Autodesk Inventor part; units mm, degrees
ref_plane "作業平面1" through (31.0675, 0, 31.152) normal (0, 1, 0) x (0, 0, 1)
ref_plane "YZ Plane" through (0, 0, 0) normal (1, 0, 0) x (0, 1, 0)
ref_plane "XZ Plane" through (0, 0, 0) normal (0, 1, 0) x (-1, 0, 0)
sketch "スケッチ1" plane through (0, 0, 0) normal (0, 1, 0) x (-1, 0, 0)
  line L0 (18, 8) -> (-18, 8) construction
  line L1 (-18, 8) -> (-18, -8) construction
  line L2 (-18, -8) -> (18, -8) construction
  line L3 (18, -8) -> (18, 8) construction
  line L4 (18, 8) -> (-18, -8) construction
  line L5 (-18, 8) -> (18, -8) construction
  circle A0 centre (18, -8) radius 1.1
  circle A1 centre (-18, -8) radius 1.1
  circle A2 centre (-18, 8) radius 1.1
  circle A3 centre (18, -8) radius 2.5
  circle A4 centre (-18, -8) radius 2.5
  circle A5 centre (-18, 8) radius 2.5
  line L6 (18, -10.5) -> (-18, -10.5)
  line L7 (-15.5, 8) -> (-15.5, -8)
  line L8 (-18, -5.5) -> (18, -5.5)
  line L9 (-20.5, -8) -> (-20.5, 8)
  line L10 (-20.5, 0) -> (18, 0) construction
  circle A6 centre (18, 8) radius 1.1
  circle A7 centre (18, 8) radius 2.5
  line L11 (18, 10.5) -> (-18, 10.5)
  line L12 (-18, 5.5) -> (18, 5.5)
  point P0 (0, 0)
  point P1 (-17.0032, -10.2927)
  point P2 (-17.0032, 10.2927)
  point P3 (-15.5, -5.5)
  point P4 (18.123, -10.497)
  point P5 (-15.5, 5.5)
  dimension "d0" = 36
  dimension "d2" = 2.2
  dimension "d3" = 2.2
  dimension "d5" = 5
  dimension "d17" = 16
extrude "押し出し1" add sketch "スケッチ1" along normal blind 1.5 contours L8 A4 L9 A5 L12 L7 | L7 A4 L8 | A4 | L12 A5 L7 | L7 A5 L11 A7 L12 | A5 | A7
fillet "フィレット1" radius 2 1 edges at (15.5, 0.75, 5.5)
sketch "スケッチ2" plane through (0, 1.5, 0) normal (0, 1, 0) x (1, 0, 0)
  line L0 (39.5, 8) -> (23.5, -8) construction
  line L1 (20.5, -8) -> (20.5, 8)
  circle A0 centre (35.0355, 3.5355) radius 1.1
  circle A1 centre (27.9645, -3.5355) radius 1.1
  line L2 (31.5, 0) -> (34.6629, -3.1629) construction
  circle A2 centre (27.9645, -3.5355) radius 2.5
  circle A3 centre (35.0355, 3.5355) radius 2.5
  line L3 (15.5, 8) -> (15.5, -3.5)
  arc A4 (18, -10.5) -> (20.5, -8) centre (18, -8) ccw
  line L4 (20.5, -8) -> (20.5, 8)
  arc A5 (20.5, 8) -> (15.5, 8) centre (18, 8) ccw
  circle A6 centre (18, 8) radius 1.1
  circle A7 centre (18, -8) radius 1.1
  line L5 (18.6338, 10.4183) -> (35.6693, 5.9539)
  line L6 (19.0222, -10.2815) -> (28.9867, -5.817)
  line L7 (36.8033, 1.7678) -> (29.7322, -5.3033)
  line L8 (13.5, -5.5) -> (-18, -5.5)
  arc A8 (-18, -5.5) -> (-18, -10.5) centre (-18, -8) ccw
  line L9 (-18, -10.5) -> (18, -10.5)
  arc A9 (13.5, -5.5) -> (15.5, -3.5) centre (13.5, -3.5) ccw
  point P0 (0, 0)
  dimension "d18" = 45
  dimension "d19" = 3
  dimension "d20" = 2.2
  dimension "d21" = 2.2
  dimension "d22" = 5
  dimension "d23" = 5
  dimension "d24" = 5
  dimension "d25" = 5
extrude "押し出し2" add sketch "スケッチ2" against normal up to surface (1.5 mm away) contours L1 A5 L5 A3 L7 A2 L6 A4 | A2 | A3
ref_plane "作業平面1" through (31.0675, 0, 31.152) normal (0, 1, 0) x (0, 0, 1)
sketch "スケッチ3" plane through (0, 1.5, 0) normal (0, 1, 0) x (1, 0, 0)
  line L0 (36.8033, 5.3033) -> (66.8553, -24.7487)
  line L1 (52.1378, -80.9663) -> (-19.4142, -9.4142)
  line L2 (51.8293, -9.7227) -> (16.3618, -45.1902) construction
  circle A0 centre (35.0355, 3.5355) radius 1.1
  circle A1 centre (27.9645, -3.5355) radius 1.1
  arc A2 (18, -10.5) -> (19.0222, -10.2815) centre (18, -8) ccw
  line L3 (19.0222, -10.2815) -> (28.9867, -5.817)
  arc A3 (28.9867, -5.817) -> (29.7322, -5.3033) centre (27.9645, -3.5355) ccw
  line L4 (29.7322, -5.3033) -> (36.8033, 1.7678)
  arc A4 (36.8033, 1.7678) -> (35.6693, 5.9539) centre (35.0355, 3.5355) ccw
  line L5 (35.6693, 5.9539) -> (18.6338, 10.4183)
  arc A5 (18.6338, 10.4183) -> (15.5, 8) centre (18, 8) ccw
  line L6 (15.5, 8) -> (15.5, -3.5)
  arc A6 (13.5, -5.5) -> (15.5, -3.5) centre (13.5, -3.5) ccw
  line L7 (13.5, -5.5) -> (-18, -5.5)
  arc A7 (-18, -5.5) -> (-18, -10.5) centre (-18, -8) ccw
  line L8 (-18, -10.5) -> (18, -10.5)
  circle A8 centre (18, -8) radius 1.1
  circle A9 centre (-18, -8) radius 1.1
  circle A10 centre (18, 8) radius 1.1
  line L9 (66.8553, -24.7487) -> (36.8033, 5.3033)
  line L10 (-19.4142, -9.4142) -> (52.1378, -80.9663)
  circle A11 centre (65.0876, -26.5165) radius 1.1
  circle A12 centre (58.0165, -33.5876) radius 1.1
  arc A13 (51.2706, -42.5298) -> (51.052, -43.552) centre (53.552, -43.552) ccw
  line L11 (51.2706, -42.5298) -> (55.735, -32.5654)
  arc A14 (56.2487, -31.8198) -> (55.735, -32.5654) centre (58.0165, -33.5876) ccw
  line L12 (56.2487, -31.8198) -> (63.3198, -24.7487)
  arc A15 (67.5059, -25.8827) -> (63.3198, -24.7487) centre (65.0876, -26.5165) ccw
  line L13 (67.5059, -25.8827) -> (71.9704, -42.9183)
  arc A16 (69.552, -46.052) -> (71.9704, -42.9183) centre (69.552, -43.552) ccw
  line L14 (69.552, -46.052) -> (58.052, -46.052)
  arc A17 (58.052, -46.052) -> (56.052, -48.052) centre (58.052, -48.052) ccw
  line L15 (56.052, -48.052) -> (56.052, -79.552)
  arc A18 (51.052, -79.552) -> (56.052, -79.552) centre (53.552, -79.552) ccw
  line L16 (51.052, -79.552) -> (51.052, -43.552)
  circle A19 centre (53.552, -43.552) radius 1.1
  circle A20 centre (53.552, -79.552) radius 1.1
  circle A21 centre (69.552, -43.552) radius 1.1
  point P0 (0, 0)
  point P1 (61.552, -61.552)
extrude "押し出し3" add sketch "スケッチ3" against normal up to surface (1.5 mm away) contours A15 L13 A16 L14 A17 L15 A18 L16 A13 L11 A14 L12
sketch "スケッチ4" plane through (0, 1.5, 0) normal (0, 1, 0) x (1, 0, 0)
  arc A0 (51.052, -79.552) -> (56.052, -79.552) centre (53.552, -79.552) ccw
  line L0 (51.7843, -81.3198) -> (-19.7678, -9.7678)
  arc A1 (-18, -5.5) -> (-18, -10.5) centre (-18, -8) ccw
  arc A2 (-18, -5.5) -> (-18, -10.5) centre (-18, -8) ccw
  arc A3 (51.052, -79.552) -> (56.052, -79.552) centre (53.552, -79.552) ccw
  circle A4 centre (53.552, -79.552) radius 2.5
  line L1 (55.3198, -77.7843) -> (-16.9645, -5.5)
  line L2 (51.052, -43.552) -> (51.052, -79.552)
  line L3 (-18, -10.5) -> (18, -10.5)
  line L4 (13.5, -5.5) -> (-18, -5.5)
  point P0 (0, 0)
  point P1 (-11.9645, -10.5)
  point P2 (51.052, -73.5165)
extrude "押し出し5" add sketch "スケッチ4" against normal up to surface (1.5 mm away) contours A0 L0 A1 L3 L1 L2
fillet "フィレット2" radius 2 2 edges at (51.052, 0.75, 73.5165) (-11.9645, 0.75, 10.5)
sketch "スケッチ5" plane through (0, 1.5, 0) normal (0, 1, 0) x (1, 0, 0)
  circle A0 centre (-11.5, 0) radius 6.2325
  circle A1 centre (61.552, -73.052) radius 6.2325
  point P0 (0, 0)
extrude "押し出し6" cut sketch "スケッチ5" against normal through all
sketch "スケッチ6" plane through (0, 1.5, 0) normal (0, 1, 0) x (1, 0, 0)
  line L0 (-7.136, -10.5) -> (18, -10.5)
  line L1 (16.3198, -10.5) -> (51.052, -45.2322)
  line L2 (51.052, -68.6881) -> (51.052, -43.552)
  line L3 (51.2706, -42.5298) -> (55.735, -32.5654)
  line L4 (51.6795, -41.6171) -> (19.935, -9.8725)
  line L5 (28.9867, -5.817) -> (19.0222, -10.2815)
  line L6 (47.6378, -70.1023) -> (-8.5503, -13.9142)
  arc A0 (18, -10.5) -> (19.0222, -10.2815) centre (18, -8) ccw
  arc A1 (51.2706, -42.5298) -> (51.052, -43.552) centre (53.552, -43.552) ccw
  point P0 (0, 0)
  dimension "d37" = 3
  dimension "d38" = 20
extrude "押し出し7" add sketch "スケッチ6" against normal up to surface (1.5 mm away)
fillet "フィレット3" radius 2 4 edges at (16.3198, 0.75, 10.5) (19.935, 0.75, 9.8725) (51.052, 0.75, 45.2322) (51.6795, 0.75, 41.6171)
sketch "スケッチ7" plane through (0, 1.5, 0) normal (0, 1, 0) x (1, 0, 0)
  arc A0 (-7.136, -10.5) -> (-8.5503, -13.9142) centre (-7.136, -12.5) ccw construction
  line L0 (-8.5503, -13.9142) -> (-12.0858, -17.4497) construction
  line L1 (-19.7678, -9.7678) -> (51.7843, -81.3198) construction
  line L2 (-10.318, -15.682) -> (45.8701, -71.8701) construction
  arc A1 (47.6378, -70.1023) -> (51.052, -68.6881) centre (49.052, -68.6881) ccw construction
  line L3 (47.6378, -70.1023) -> (44.1023, -73.6378) construction
  circle A2 centre (0.2886, -26.2886) radius 1.1
  line L4 (47.6378, -70.1023) -> (-8.5503, -13.9142)
  line L5 (17.776, -43.776) -> (16.0083, -45.5438) construction
  circle A3 centre (35.2635, -61.2635) radius 1.1
  point P0 (0, 0)
  dimension "d42" = 2.2
  dimension "d43" = 15
extrude "押し出し8" cut sketch "スケッチ7" against normal through all
equation "\"d23\" = d22"
equation "\"d24\" = d25"
equation "\"d26\" = d22"
properties part number "piti_mata"
Source: CAD feature listing. Evaluate the final solid. Frame: model axes, mm. A direction names the side the tool comes from. Give positions to 0.01 mm unless a question says otherwise; leave off trailing zeros. Write each loop counter-clockwise with the first axis right and the second up, starting at its lowest first coordinate (ties: lowest second). Pieces come first, ordered by that corner, then holes. Notation, with made-up numbers: (-39, 40) - (-10, 40) arc R30 cw to (-10, 62) - close; hole circle Ø3 at (-12.75, 84). An arc over 180 degrees is marked (long way). One line per item, written item: value. Start each with the question number.
Q1. Material intervals for probe 1 along X at (y, z) = (1.2, 44); probe 2 along X at (y, z) = (0.5, 36.5); probe 3 along Z at (x, y) = (37, 0.1), sorted ascending. Write a range as from..to.
Q2. Set-up query: faces 5 (the face through (54.28, 0.76, 35.81)), 6 (the face through (33.317, 0.76, 1.718)), 7 (the face through (33.45, 0.76, 27.63)), 8 (the face through (27.03, 0.76, -8.22)). Return all of +Z, -Z, +X, -X, +Y, -Y with unobstructed straight access to the full face (end or side cutting, diameter ignored); none if empty.
Q3. Section query A-A, the plane x = 3. Return the cut outline in (y, z).
Q4. Section query C-C, the plane x = 40.5. Return the cut outline in (y, z).
Q5. Section query D-D, the plane z = 74. Return the cut outline in (x, y).
Q6. Section query B-B, the plane y = 0.35. Count the separate pieces of the cut face and the enclosed holes in it, then the cut area to 3 significant figures.
Q7. Draft query along X for faces 1 (the face through (59.735, 0.76, 28.334)), 2 (the face through (71.511, 0.76, 45.105)), 3 (the face through (36, 1.5, 29)), 4 (the face through (36, 0.76, 25.94)). Return one class per face: +X half, -X half, draft (parallel to the pull), parting line (faces both ways), or undercut.
Answer:
1. probe 1: x = 14.46..21.54, 49.82..52.55, 54.56..68.55, 70.56..72.01
1. probe 2: x = 6.96..14.04, 42.32..46.56, 53.97..70.29
1. probe 3: z = -5.08..-1.99, 26.94..31.18, 59.46..66.54
2. face 5: -Z, +Y, -Y
2. face 6: +X, +Y, -Y
2. face 7: +Y, -Y
2. face 8: -Z, +X, +Y, -Y
3. outline: (0, 5.5) - (1.5, 5.5) - (1.5, 10.5) - (0, 10.5) - close; (0, 25.46) - (1.5, 25.46) - (1.5, 32.54) - (0, 32.54) - close
4. outline: (0, 30.44) - (1.5, 30.44) - (1.5, 34.68) - (0, 34.68) - close; (0, 62.96) - (1.5, 62.96) - (1.5, 70.04) - (0, 70.04) - close
5. outline: (44.46, 0) - (55.39, 0) - (55.39, 1.5) - (44.46, 1.5) - close
6. separate pieces: 1
6. enclosed holes: 13
6. area: 1,560 mm2
7. face 1: undercut
7. face 2: +X half
7. face 3: draft
7. face 4: undercut
